Model file for the job. Use its own axes, mm. Face numbers are marked on the shaded views. A direction names the side the tool comes from. Give positions to 0.01 mm unless a question says otherwise; leave off trailing zeros. Order: outer loops, then holes, each group sorted by start corner. A loop starts at its lowest first (then second) coordinate and runs counter-clockwise, first axis right, second up. Notation, with made-up numbers: (24, 7) - (50, 7) arc R9 cw to (50, 13) - close; hole circle Ø1 at (52, 20). An arc over 180 degrees is marked (long way). Return JSON: item names as keys, results as strings. Group by question number.
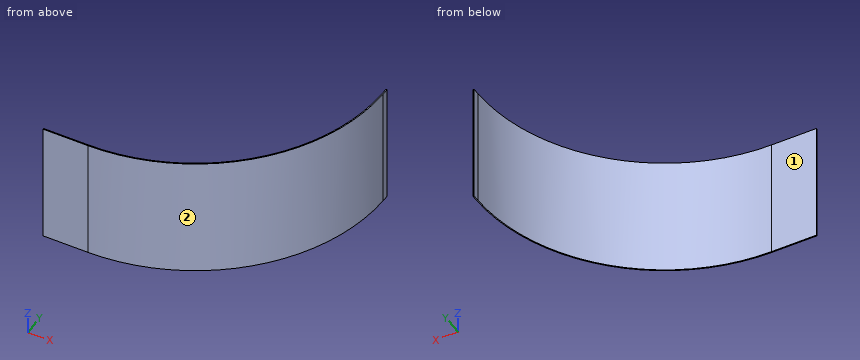
from build123d import *

# Parameters (mm, degrees)
EXTRUDE_THIN1_DEPTH = 670


with BuildPart() as part:
    # Sketch1 → Extrude-Thin1 (new body)
    with BuildSketch(Plane.XY):
        with BuildLine():
            Line((2235, -4410), (2235, -4450))
            ThreePointArc((2235, -4450), (1931.855518528, -5181.855518528), (1200, -5485))
            Line((1200, -5485), (950, -5485))
            Line((950, -5485), (950, -5491))
            Line((950, -5491), (1200, -5491))
            ThreePointArc((1200, -5491), (1936.098159215, -5186.098159215), (2241, -4450))
            Line((2241, -4450), (2241, -4410))
            Line((2241, -4410), (2235, -4410))
        make_face()
    extrude(amount=-EXTRUDE_THIN1_DEPTH)


solid = part.part
(1) Drop flat-ended pins along their axis: pin 1 Ø1 at (y, z) = (-4609, -395) entering from +X; pin 2 Ø1 at (x, z) = (1745.5, -106) entering from +Y; pin 3 Ø8 at (x, z) = (1900, -130) entering from +Y. Give the stop position or say it passes through.
(2) Drill centre lines: L1, parallel to Y at x = 1036, z = -183; L2, parallel to X at y = -5144.5, z = -433.5; L3, parallel to X at y = -4651, z = -416. Where is each one in solid material? Low to high.
(3) Slice it at A-A (z = -615.5). Give the cut face in (x, y).
(4) 3-axis set-ups, long thin cutter, end or side, ignore diameter. For the marked faces 1 and 2: which of +Z, -Z, +X, -X, +Y, -Y reach the whole face in a straight line?
(5) Slice it at C-C (y = -5018.5). Give the cut face in (x, z), and give its area (3 significant figures).
(6) Slice it at B-B (x = 1089). Give the cut face in (y, z).
Result set:
{
 "1": {"pin 1": "stops at x = 2228.86", "pin 2": "stops at y = -5329.27", "pin 3": "stops at y = -5208.69"},
 "2": {"L1": "y = -5491 to -5485", "L2": "x = 1967.39 to 1975.47", "L3": "x = 2215.3 to 2221.41"},
 "3": {"outline": "(950, -5491) - (1200, -5491) arc R1041 ccw to (2241, -4450) - (2241, -4410) - (2235, -4410) - (2235, -4450) arc R1035 cw to (1200, -5485) - (950, -5485) - close"},
 "4": {"face 1": "+Z, -Z, -X, +Y", "face 2": "+Z, -Z, +X, -Y"},
 "5": {"outline": "(2064.89, -670) - (2072.06, -670) - (2072.06, 0) - (2064.89, 0) - close", "area": "4,800 mm²"},
 "6": {"outline": "(-5491, -670) - (-5485, -670) - (-5485, 0) - (-5491, 0) - close"}
}
